Geometry check sheet. Reference: the model listing, model coordinates, mm. A direction names the side the tool comes from. Coordinates: 2 decimals unless noted, no trailing zeros. Order: outer loops, then holes, each group sorted by start corner. A loop starts at its lowest first (then second) coordinate and runs counter-clockwise, first axis right, second up. Notation, with made-up numbers: (-1.75, 63.25) - (22.25, 63.25) arc R21 cw to (22.25, 93.25) - close; hole circle Ø4 at (49.5, 64). An arc over 180 degrees is marked (long way). Return JSON: item names as keys, results as strings. Group by question number.
Item 1: Scan lines: probe 1 along X at (y, z) = (203.2, 135); probe 2 along X at (y, z) = (-200, 118); probe 3 along X at (y, z) = (-349, 23). Record each from-to range of solid material in increasing order.
Item 2: Draft check along X on faces 1 (the flat face through (200.66, -6, 120)), 2 (the cylindrical face through (-10.746, 121.352, 108.174)), 3 (the flat face through (-200.66, -6, 120)), 4 (the flat face through (-19, -142, 0)). Enter one of: pulls with the +X half, pulls with the -X half, needs draft (parallel to the pull), parting line crosses it, or undercut.
Item 3: Section check C-C on y = 304.8. Enter the section's corners in (x, z).
Item 4: Gauge pin test, flat end, axial feed: pin 1 (5 mm diameter, centred on x = 145.5, y = -202.5, fed in from -Z). Record the tip position at first contact, or that the pin passes through.
Item 5: Section check A-A on z = 66. Enter the section's corners in (x, y).
Item 6: Section check D-D on y = -203.2. Enter the section's corners in (x, z), then the cut area to 3 significant figures.
Item 7: Tool access check on faces 5 (the flat face through (-19, 264, 0)), 6 (the flat face through (170.18, 5, 105)), 7 (the cylindrical face through (93.66, 365.24, 266.38)). Record the directions out of +Z, -Z, +X, -X, +Y, -Y that give a thin tool (end or side, any length) a straight path to the whole face; none if there is none.
from build123d import *

# Parameters (mm, degrees)
F0_W     = 401.32
F0_H     = 807.72
F1_DEPTH = 243.84
F2_R     = 60.96
F3_DEPTH = 45.72
F4_W     = 340.36
F4_H     = 746.76
F5_DEPTH = 213.36
F6_R     = 82.55
F6_R_2   = 63.178676
F7_DEPTH = 213.36


with BuildPart() as f1:
    # F0 (on Top) → F1 (new body)
    with BuildSketch(Plane.XY):
        Rectangle(F0_W, F0_H)
    extrude(amount=F1_DEPTH)

    # F2 (on face) → F3 (join)
    with BuildSketch(Plane.XY.offset(243.84)):
        with Locations((101.6, 304.8)):
            Circle(F2_R)
        with Locations((101.6, 101.6)):
            Circle(F2_R)
        with Locations((101.6, -101.6)):
            Circle(F2_R)
        with Locations((101.6, -304.8)):
            Circle(F2_R)
        with Locations((-101.6, 304.8)):
            Circle(F2_R)
        with Locations((-101.6, 101.6)):
            Circle(F2_R)
        with Locations((-101.6, -101.6)):
            Circle(F2_R)
        with Locations((-101.6, -304.8)):
            Circle(F2_R)
    extrude(amount=F3_DEPTH)

    # F4 (on face) → F5 (cut)
    with BuildSketch(Plane(origin=(0, 0, 0), x_dir=(1, 0, 0), z_dir=(0, 0, -1))):
        Rectangle(F4_W, F4_H)
    extrude(amount=-F5_DEPTH, mode=Mode.SUBTRACT)

    # F6 (on face) → F7 (join)
    with BuildSketch(Plane(origin=(0, 0, 213.36), x_dir=(1, 0, 0), z_dir=(0, 0, -1))):
        Circle(F6_R)
        Circle(F6_R_2, mode=Mode.SUBTRACT)
        with Locations((0, 203.2)):
            Circle(F6_R)
        with Locations((0, 203.2)):
            Circle(F6_R_2, mode=Mode.SUBTRACT)
        with Locations((0, -203.2)):
            Circle(F6_R)
        with Locations((0, -203.2)):
            Circle(F6_R_2, mode=Mode.SUBTRACT)
    extrude(amount=F7_DEPTH)


solid = f1.part
Computed:
{
 "1": {"probe 1": "x = -200.66 to -170.18, -82.55 to -63.18, 63.18 to 82.55, 170.18 to 200.66", "probe 2": "x = -200.66 to -170.18, -82.49 to -63.1, 63.1 to 82.49, 170.18 to 200.66", "probe 3": "x = -200.66 to -170.18, 170.18 to 200.66"},
 "2": {"face 1": "pulls with the +X half", "face 2": "undercut", "face 3": "pulls with the -X half", "face 4": "needs draft"},
 "3": {"outline": "(-200.66, 0) - (-170.18, 0) - (-170.18, 213.36) - (170.18, 213.36) - (170.18, 0) - (200.66, 0) - (200.66, 243.84) - (162.56, 243.84) - (162.56, 289.56) - (40.64, 289.56) - (40.64, 243.84) - (-40.64, 243.84) - (-40.64, 289.56) - (-162.56, 289.56) - (-162.56, 243.84) - (-200.66, 243.84) - close"},
 "4": {"pin 1": "stops at z = 213.36"},
 "5": {"outline": "(-200.66, -403.86) - (200.66, -403.86) - (200.66, 403.86) - (-200.66, 403.86) - close; circle Ø165.1 at (0, -203.2); circle Ø165.1 at (0, 0); circle Ø165.1 at (0, 203.2); hole (-170.18, -373.38) - (170.18, -373.38) - (170.18, 373.38) - (-170.18, 373.38) - close; hole circle Ø126.36 at (0, -203.2); hole circle Ø126.36 at (0, 0); hole circle Ø126.36 at (0, 203.2)"},
 "6": {"outline": "(-200.66, 0) - (-170.18, 0) - (-170.18, 213.36) - (-82.55, 213.36) - (-82.55, 0) - (-63.18, 0) - (-63.18, 213.36) - (63.18, 213.36) - (63.18, 0) - (82.55, 0) - (82.55, 213.36) - (170.18, 213.36) - (170.18, 0) - (200.66, 0) - (200.66, 243.84) - (-200.66, 243.84) - close", "area": "33,500 mm²"},
 "7": {"face 5": "-Z, +X, -X, +Y, -Y", "face 6": "-Z", "face 7": "+Z"}
}
